```python
from build123d import *

# Parameters (mm, degrees)
SKETCH_5_W          = 24
SKETCH_5_H          = 15
EXTRUDE_5_DEPTH     = 5
CUT_EXTRUDE_6_REACH = 30.74
SKETCH_6_R          = 2.6
SKETCH_7_W          = 6
SKETCH_7_H          = 15
EXTRUDE_7_DEPTH     = 40
SKETCH_8_R          = 2.6
CUT_EXTRUDE_8_DEPTH = 54.16013544


with BuildPart() as part:
    # Эскиз5 → Вытянуть5 (new body)
    with BuildSketch(Plane(origin=(0, 0, 0), x_dir=(1, 0, 0), z_dir=(0, 1, 0))):
        with Locations((12, 7.5)):
            Rectangle(SKETCH_5_W, SKETCH_5_H)
    extrude(amount=EXTRUDE_5_DEPTH)

    # Эскиз6 → Вытянуть6 (cut, up to next)
    with BuildSketch(Plane(origin=(0, 5, 0), x_dir=(1, 0, 0), z_dir=(0, 1, 0)), mode=Mode.PRIVATE) as cut_extrude_6_sk1:
        with Locations(Location((12, 7.5, 0), (0, 0, 270))):
            Circle(SKETCH_6_R)
    cut_extrude_6_tool1 = extrude(cut_extrude_6_sk1.sketch, amount=-CUT_EXTRUDE_6_REACH, mode=Mode.PRIVATE) & part.part
    add(cut_extrude_6_tool1.solids().sort_by_distance((12, 5, -7.5))[0], mode=Mode.SUBTRACT)

    # Эскиз7 → Вытянуть7 (add)
    with BuildSketch(Plane(origin=(0, 5, 0), x_dir=(1, 0, 0), z_dir=(0, 1, 0))):
        with Locations((3, 7.5)):
            Rectangle(SKETCH_7_W, SKETCH_7_H)
        with Locations((21, 7.5)):
            Rectangle(SKETCH_7_W, SKETCH_7_H)
    extrude(amount=EXTRUDE_7_DEPTH)

    # Эскиз8 → Вытянуть8 (cut, through all)
    with BuildSketch(Plane.ZY):
        with Locations((-7.5, 20)):
            Circle(SKETCH_8_R)
    extrude(amount=-CUT_EXTRUDE_8_DEPTH, mode=Mode.SUBTRACT)


solid = part.part
```
Could you check a few things on this model? Use its own coordinates, in mm. A direction names the side the tool comes from. Round coordinates to 2 decimals unless told otherwise and drop trailing zeros. Write each loop counter-clockwise with the first axis right and the second up, starting at its lowest first coordinate (ties: lowest second). Pieces come first, ordered by that corner, then holes. Notation, with made-up numbers: M -7.75,-4.75 L 37.25,-4.75 A19 ccw 37.25,0.25 Z; hole C 73,-22.5 d8. An arc over 180 degrees is marked long. Write each question's results on one line, items separated by ' | '. Start each with the question number.
1. Imagine slicing it at B-B on y = 20. List the corners of the cut face in (x, z) for me.
2. Imagine slicing it at A-A on z = -7.5. List the corners of the cut face in (x, y) for me.
3. Thinking about a two-plate mould opening in Z: for faces 1 (the face through (20, 22, -15)), 2 (the face through (18, 25, -7)), 3 (the face through (2.958, 22.578, -7.838)), 4 (the face through (20, 22, 0)), which applies, +Z half, -Z half, draft (parallel to the pull), parting line (faces both ways), or undercut?
4. I'm going to push a flat-ended pin straight in: pin 1 Ø6 at (x, z) = (12, -7.5) entering from +Y. Where does the tip first touch, or does it pass through?
5. Imagine slicing it at D-D on y = 32. List the corners of the cut face in (x, z) for me, and give its area (3 significant figures).
6. Imagine slicing it at C-C on x = 12. List the corners of the cut face in (y, z) for me.
7. I need wall thicknesses on L1, parallel to X at y = 9, z = -10.25; L2, parallel to Y at x = 4.35, z = -7.5; L3, parallel to X at y = 2.8, z = -7.5. Which ranges of each line are inside material? Lowest first, please. Write a range as from..to.
8. On a 3-axis mill with a long thin cutter (end or side, diameter ignored), from which of +Z, -Z, +X, -X, +Y, -Y can I reach the whole of each face in a straight line? I mean faces 5 (the face through (6, 25, -7)), 6 (the face through (24, 22.2, -5.7)). Say none if no direction works.
Result sheet:
1) outline: M 0,-15 L 6,-15 L 6,-10.1 L 0,-10.1 Z; M 0,-4.9 L 6,-4.9 L 6,0 L 0,0 Z; M 18,-15 L 24,-15 L 24,-10.1 L 18,-10.1 Z; M 18,-4.9 L 24,-4.9 L 24,0 L 18,0 Z
2) outline: M 0,0 L 9.4,0 L 9.4,5 L 6,5 L 6,17.4 L 0,17.4 Z; M 0,22.6 L 6,22.6 L 6,45 L 0,45 Z; M 14.6,0 L 24,0 L 24,17.4 L 18,17.4 L 18,5 L 14.6,5 Z; M 18,22.6 L 24,22.6 L 24,45 L 18,45 Z
3) face 1: -Z half | face 2: draft | face 3: undercut | face 4: +Z half
4) pin 1: stops at y = 5
5) outline: M 0,-15 L 6,-15 L 6,0 L 0,0 Z; M 18,-15 L 24,-15 L 24,0 L 18,0 Z | area: 180 mm^2
6) outline: M 0,-15 L 5,-15 L 5,-10.1 L 0,-10.1 Z; M 0,-4.9 L 5,-4.9 L 5,0 L 0,0 Z
7) L1: x = 0..6, 18..24 | L2: y = 0..17.4, 22.6..45 | L3: x = 0..9.4, 14.6..24
8) face 5: +Z, -Z, +Y | face 6: +Z, -Z, +X, +Y, -Y
